Design review of the part shown in the three views and the two pictorial views. Dimensions are in mm from the part's minimum x, y and z. A direction names the side the tool comes from. Round coordinates to 2 decimals unless told otherwise and drop trailing zeros. Loops run counter-clockwise (first coordinate to the right, second up) from the corner with the lowest first, then second, coordinate; pieces in that order, holes last.
1. Draft analysis for pull direction X (two halves, no side actions). For the marked faces 1, 2 and 3, state which applies: released by +X, released by -X, zero draft, split by the parting line, or undercut.
2. To check wall thickness, follow line 1 along Z through (x, y) = (66.5, 79.5); line 2 along Y through (x, z) = (92, 19) (1 decimal); line 3 along Y through (x, z) = (32, 40.5) (1 decimal). State the ranges of each line that lie inside material, in increasing order.
3. Consider section C-C on y = 22. State the section outline as (x, z) points (1 decimal), then the cut area to 3 significant figures.
4. Consider section B-B on y = 50. State the section outline as (x, z) points (1 decimal), then the cut area to 3 significant figures.
5. Consider section D-D on z = 16. State the section outline as (x, y) points (1 decimal).
6. Clearance check with flat-ended pins moving along their axes: pin 1 Ø20 at (x, z) = (32, 40.5) entering from -Y; pin 2 Ø14.5 at (y, z) = (25.5, 38) entering from -X (1 decimal); pin 3 Ø1 at (y, z) = (18.5, 15.5) entering from +X. State where each tip first meets the part, or that it passes through.
7. Tool access review of the marked faces 4 and 5: name each direction out of +Z, -Z, +X, -X, +Y, -Y from which nothing blocks a thin tool from reaching the whole face with its end or side.
8. Consider section A-A on x = 14. State the section outline as (y, z) points (1 decimal).
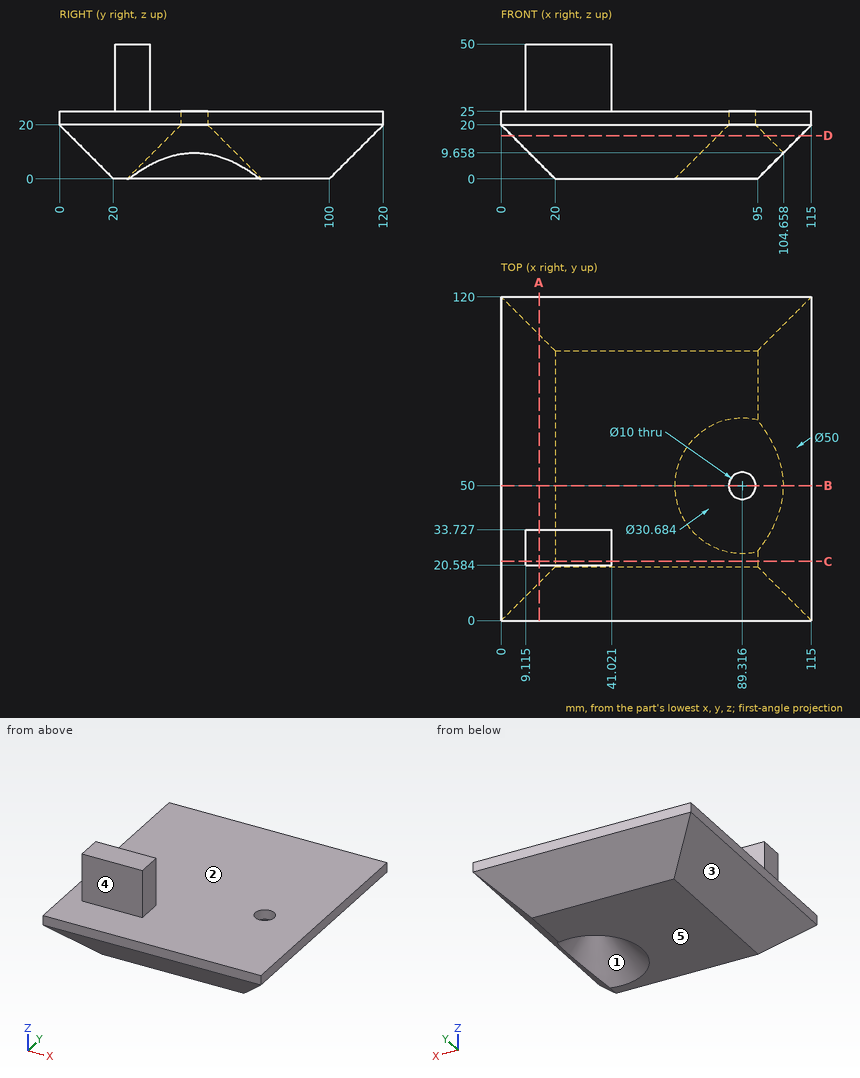
Resolved:
1. face 1: undercut
1. face 2: zero draft
1. face 3: released by -X
2. line 1: z = 0 to 25
2. line 2: y = 1 to 44.6, 55.4 to 119
2. line 3: y = 20.6 to 33.7
3. outline: (0, 20) - (20, 0) - (95, 0) - (115, 20) - (115, 25) - (41, 25) - (41, 50) - (9.1, 50) - (9.1, 25) - (0, 25) - close
3. area: 3,270 mm2
4. outline: (0, 20) - (20, 0) - (64.3, 0) - (84.3, 20) - (84.3, 25) - (0, 25) - close; (94.3, 20) - (104.7, 9.7) - (115, 20) - (115, 25) - (94.3, 25) - close
4. area: 1,920 mm2
5. outline: (4, 4) - (111, 4) - (111, 116) - (4, 116) - close; hole circle Ø18 at (89.3, 50)
6. pin 1: stops at y = 20.58
6. pin 2: stops at x = 9.1
6. pin 3: stops at x = 111
7. face 4: +Z, +X, -X, -Y
7. face 5: -Z, +X, -X, +Y, -Y
8. outline: (0, 20) - (14, 6) - (106, 6) - (120, 20) - (120, 25) - (33.7, 25) - (33.7, 50) - (20.6, 50) - (20.6, 25) - (0, 25) - close
